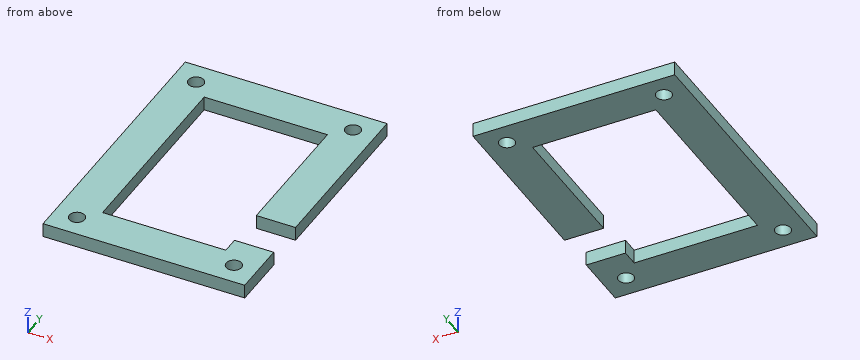
Autodesk Inventor part; units mm, degrees
ref_plane "YZ Plane" through (0, 0, 0) normal (1, 0, 0) x (0, 1, 0)
ref_plane "XZ Plane" through (0, 0, 0) normal (0, 1, 0) x (-1, 0, 0)
ref_plane "XY Plane" through (0, 0, 0) normal (0, 0, 1) x (1, 0, 0)
ref_plane "Plano de trabajo1" through (0, 0, 0) normal (0, 0, 1) x (1, 0, 0)
sketch "Boceto1" plane through (0, 0, 0) normal (0, 0, 1) x (1, 0, 0)
  line L0 (-22, -35) -> (22, -35)
  line L1 (-22, 35) -> (-22, -35)
  line L2 (22, 35) -> (-22, 35)
  line L3 (22, -35) -> (22, 35)
  line L4 (-36, -49) -> (36, -49)
  line L5 (36, -49) -> (36, 49)
  line L6 (36, 49) -> (-36, 49)
  line L7 (-36, 49) -> (-36, -49)
  line L8 (-36, -49) -> (36, -49)
  line L9 (36, -49) -> (36, 49)
  line L10 (36, 49) -> (-36, 49)
  line L11 (-36, 49) -> (-36, -49)
  line L12 (-22, -35) -> (22, -35)
  line L13 (22, 35) -> (-22, 35)
  line L14 (-22, 35) -> (-22, -35)
  circle A0 centre (28, -41) radius 2.75
  circle A1 centre (-28, 41) radius 2.75
  circle A2 centre (28, 41) radius 2.75
  circle A3 centre (-28, -41) radius 2.75
  line L15 (36, -49) -> (36, -29)
  line L16 (36, -29) -> (22, -29)
  line L17 (36, -29) -> (36, -14)
  line L18 (36, -14) -> (22, -14)
  line L19 (22, -35) -> (22, -29)
  line L20 (22, -14) -> (22, 35)
  point P0 (0, 0)
  dimension "d16" = 20
  dimension "d17" = 15
  dimension "d18" = 0
ref_plane "Plano de trabajo4" through (0, 0, 5) normal (0, 0, 1) x (1, 0, 0)
ref_plane "Plano de trabajo3" through (0, 0, 5) normal (0, 0, 1) x (1, 0, 0)
ref_plane "Plano de trabajo2" through (0, 0, 5) normal (0, 0, 1) x (1, 0, 0)
sketch "Boceto4" plane through (0, 0, 5) normal (0, 0, 1) x (1, 0, 0)
  point P0 (0, 0)
extrude "Extrusión2" add sketch "Boceto1" along normal blind 5 contours L0 L3 L16 L5 L4 L7 L6 L18 L2 L1
sketch "Boceto2" plane through (0, 0, 5) normal (0, 0, 1) x (1, 0, 0)
  point P0 (-28, 41)
  point P1 (28, 41)
  point P2 (28, -41)
  point P3 (-28, -41)
sketch "Boceto3" plane through (0, 0, 5) normal (0, 0, 1) x (1, 0, 0)
  point P0 (-28, 41)
  point P1 (28, 41)
  point P2 (28, -41)
  point P3 (-28, -41)
Input: part model. Units: mm. Frame: model coordinates. Give positions to 0.01 mm unless a question says otherwise; leave off trailing zeros. Write each loop counter-clockwise with the first axis right and the second up, starting at its lowest first coordinate (ties: lowest second). Pieces come first, ordered by that corner, then holes.
Q1. Section A-A, the plane x = -1.5. Output: boundary loops of the cut face in (y, z).
Q2. Section B-B, the plane y = 41. Output: boundary loops of the cut face in (x, z), plus the area to 3 significant figures.
Q3. First-contact query: P1, Ø8, axis at x = 26.5, y = 8, coming from the -Z side; P2, Ø10, axis at x = 18, y = -23, coming from the +Z side. Flat tips, straight axial feed; report the tip coordinate or a pass-through.
Q4. Material intervals for probe 1 along Y at (x, z) = (-28, 2.5); probe 2 along Y at (x, z) = (28, 2.05); probe 3 along X at (y, z) = (17.5, 0.8), sorted ascending.
Q5. Section D-D, the plane y = 29. Output: boundary loops of the cut face in (x, z).
Q6. Section C-C, the plane x = -28. Output: boundary loops of the cut face in (y, z).
Filled in:
1. outline: (-49, 0) - (-35, 0) - (-35, 5) - (-49, 5) - close; (35, 0) - (49, 0) - (49, 5) - (35, 5) - close
2. outline: (-36, 0) - (-30.75, 0) - (-30.75, 5) - (-36, 5) - close; (-25.25, 0) - (25.25, 0) - (25.25, 5) - (-25.25, 5) - close; (30.75, 0) - (36, 0) - (36, 5) - (30.75, 5) - close
2. area: 305 mm2
3. P1: stops at z = 0
3. P2: passes through
4. probe 1: y = -49 to -43.75, -38.25 to 38.25, 43.75 to 49
4. probe 2: y = -49 to -43.75, -38.25 to -29, -14 to 38.25, 43.75 to 49
4. probe 3: x = -36 to -22, 22 to 36
5. outline: (-36, 0) - (-22, 0) - (-22, 5) - (-36, 5) - close; (22, 0) - (36, 0) - (36, 5) - (22, 5) - close
6. outline: (-49, 0) - (-43.75, 0) - (-43.75, 5) - (-49, 5) - close; (-38.25, 0) - (38.25, 0) - (38.25, 5) - (-38.25, 5) - close; (43.75, 0) - (49, 0) - (49, 5) - (43.75, 5) - close
